Read the model definition and answer for the solid it produces. Units are mm, in the model's axes. A direction names the side the tool comes from. Give positions to 0.01 mm unless a question says otherwise; leave off trailing zeros. Order: outer loops, then holes, each group sorted by start corner. A loop starts at its lowest first (then second) coordinate and runs counter-clockwise, first axis right, second up. Notation, with made-up numbers: (73, 81.25) - (89, 81.25) arc R20 ccw to (89, 120.25) - close; hole circle Ø11 at (63, -15.5). An arc over 180 degrees is marked (long way). Write each question's results on one line, items separated by ' | '. Start each with the question number.
Q1. A tool of negligible diameter and unlimited length cuts with its end or side. For faces 4 (the face through (0, 2, -5)), 5 (the face through (-3.5, 1.23, 1.55)), from which of +Z, -Z, +X, -X, +Y, -Y can it reach the whole face along a straight path? Write none if from no direction.
Q2. Find the intervals of material crossed by line 1 along X through (y, z) = (3.65, 0); line 2 along Z through (x, y) = (-2.5, 0.9); line 3 along X through (y, z) = (2.55, -0.5), in increasing order. Write a range as from..to.
Q3. Find section C-C on y = 3.55. Give the vertices of the cut face in (x, z), and give its area (3 significant figures).
Q4. Find section D-D on x = -3. Give the vertices of the cut face in (y, z), and give its area (3 significant figures).
Q5. For a pull along X with two mould halves and no side action, classify faces 1 (the face through (0, 2, 5)), 2 (the face through (-5, 3, 0)), 3 (the face through (0.582, 1.232, -1.624)) as +X half, -X half, draft (parallel to the pull), parting line (faces both ways), or undercut.
Q6. Find section B-B on y = 2.1. Give the vertices of the cut face in (x, z).
Q7. Find section A-A on z = 0. Give the vertices of the cut face in (x, y), and give its area (3 significant figures).
from build123d import *

# Parameters (mm, degrees)
BASEWITH_ALIGNMENT_W = 10
BASEWITH_ALIGNMENT_H = 10
BOSS_EXTRUDE1_DEPTH  = 5
SKETCH1_R            = 0.762
SKETCH1_R_2          = 0.3
CUT_EXTRUDE6_DEPTH   = 9.660254038
CUT_EXTRUDE7_DEPTH   = 2.5
SKETCH2_W            = 10
SKETCH2_H            = 0.5
CUT_EXTRUDE8_DEPTH   = 2.5


with BuildPart() as part:
    # BaseWith Alignment → Boss-Extrude1 (new body)
    with BuildSketch(Plane(origin=(0, 0, 0), x_dir=(1, 0, 0), z_dir=(0, 1, 0))):
        Rectangle(BASEWITH_ALIGNMENT_W, BASEWITH_ALIGNMENT_H)
    extrude(amount=BOSS_EXTRUDE1_DEPTH)

    # Sketch1 → Cut-Extrude6 (cut, through all)
    with BuildSketch(Plane(origin=(0, 0, 0), x_dir=(-1, 0, 0), z_dir=(0, -1, 0))):
        with Locations(Location((0.5, 0, 0), (0, 0, 90))):
            Circle(SKETCH1_R)
        with Locations(Location((3, 0, 0), (0, 0, 90))):
            Circle(SKETCH1_R_2)
        with Locations(Location((-3, 0, 0), (0, 0, 90))):
            Circle(SKETCH1_R_2)
    extrude(amount=-CUT_EXTRUDE6_DEPTH, mode=Mode.SUBTRACT)

    # Sketch1<3> → Cut-Extrude7 (cut)
    with BuildSketch(Plane(origin=(0, 0, 0), x_dir=(-1, 0, 0), z_dir=(0, -1, 0))):
        with BuildLine():
            Line((2.017857143, -1.961432458), (-3.110714286, -1.296526148))
            ThreePointArc((-3.110714286, -1.296526148), (-4.25, 0), (-3.110714286, 1.296526148))
            Line((-3.110714286, 1.296526148), (2.017857143, 1.961432458))
            ThreePointArc((2.017857143, 1.961432458), (4.25, 0), (2.017857143, -1.961432458))
        make_face()
    extrude(amount=-CUT_EXTRUDE7_DEPTH, mode=Mode.SUBTRACT)

    # Sketch2 → Cut-Extrude8 (cut)
    with BuildSketch(Plane.XZ):
        Rectangle(SKETCH2_W, SKETCH2_H)
    extrude(amount=-CUT_EXTRUDE8_DEPTH, mode=Mode.SUBTRACT)


solid = part.part
Working result:
1) face 4: -Z, +X, -X, +Y, -Y | face 5: -Y
2) line 1: -5..-3.3, -2.7..-1.26, 0.26..2.7, 3.3..5 | line 2: -5..-1.96, 1.96..5 | line 3: -5..-1.08, 0.08..5
3) outline: (-5, -5) - (5, -5) - (5, 5) - (-5, 5) - close; hole circle Ø0.6 at (-3, 0); hole circle Ø1.52 at (-0.5, 0); hole circle Ø0.6 at (3, 0) | area: 97.6 mm²
4) outline: (0, -5) - (5, -5) - (5, -0.3) - (2.5, -0.3) - (2.5, -1.84) - (0, -1.84) - close; (0, 1.84) - (2.5, 1.84) - (2.5, 0.3) - (5, 0.3) - (5, 5) - (0, 5) - close | area: 39.3 mm²
5) face 1: draft | face 2: -X half | face 3: undercut
6) outline: (-5, -5) - (5, -5) - (5, -0.25) - (4.23, -0.25) arc R1.31 cw to (3.11, -1.3) - (-2.02, -1.96) arc R1.98 cw to (-4.23, -0.25) - (-5, -0.25) - close; (-5, 0.25) - (-4.23, 0.25) arc R1.98 cw to (-2.02, 1.96) - (3.11, 1.3) arc R1.31 cw to (4.23, 0.25) - (5, 0.25) - (5, 5) - (-5, 5) - close
7) outline: (-5, 2.5) - (-3.3, 2.5) - (-3.3, 5) - (-5, 5) - close; (-2.7, 2.5) - (-1.26, 2.5) - (-1.26, 5) - (-2.7, 5) - close; (0.26, 2.5) - (2.7, 2.5) - (2.7, 5) - (0.26, 5) - close; (3.3, 2.5) - (5, 2.5) - (5, 5) - (3.3, 5) - close | area: 18.2 mm²
